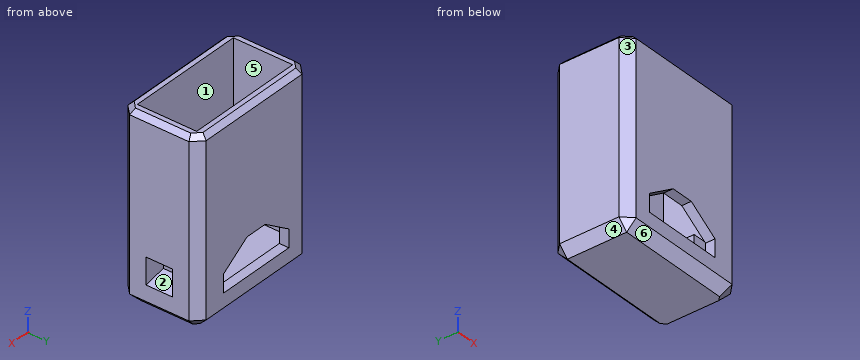
from build123d import *

# Parameters (mm, degrees)
F0_W      = 29
F0_H      = 16.5
F1_DEPTH  = 38.5
F2_T      = -2
F3_DEPTH  = 2.25
F4_SIZE   = 2
F5_SIZE   = 2
F6_SIZE   = 1
F8_DEPTH  = 16.501
F9_W      = 7.54
F9_H      = 7.25
F9_R      = 1.1
F10_DEPTH = 6.35
F11_W     = 5.538
F11_H     = 5.533
F13_W     = 5.538
F13_H     = 4.583


with BuildPart() as f1:
    # F0 (on Top) → F1 (new body)
    with BuildSketch(Plane.XY):
        with Locations((14.5, 8.25)):
            Rectangle(F0_W, F0_H)
    extrude(amount=F1_DEPTH)

    # F2
    f2_openings = [f1.faces().sort_by_distance(p)[0] for p in [
        (14.5, 8.25, 38.5),
    ]]
    offset(amount=F2_T, openings=f2_openings)

    # F3 (add): a face of the model
    f3_faces = [f1.faces().sort_by_distance(p)[0] for p in [
        (14.5, 8.25, 2),
    ]]
    extrude(f3_faces, amount=F3_DEPTH)

    # F4
    f4_edges = [f1.edges().sort_by_distance(p)[0] for p in [
        (29, 0, 19.25),
        (29, 16.5, 19.25),
    ]]
    chamfer(f4_edges, length=F4_SIZE)

    # F5
    f5_edges = [f1.edges().sort_by_distance(p)[0] for p in [
        (0, 16.5, 19.25),
        (0, 0, 19.25),
        (13.5, 16.5, 0),
        (13.5, 0, 0),
        (28, 1, 0),
        (0, 8.25, 0),
        (29, 8.25, 0),
        (28, 15.5, 0),
    ]]
    chamfer(f5_edges, length=F5_SIZE)

    # F6
    f6_edges = [f1.edges().sort_by_distance(p)[0] for p in [
        (0, 8.25, 38.5),
        (1, 1, 38.5),
        (14.5, 0, 38.5),
        (1, 15.5, 38.5),
        (14.5, 16.5, 38.5),
        (28, 15.5, 38.5),
        (29, 8.25, 38.5),
        (28, 1, 38.5),
    ]]
    chamfer(f6_edges, length=F6_SIZE)

    # F7 (on face) → F8 (cut, through all)
    with BuildSketch(Plane(origin=(0, 16.5, 0), x_dir=(-1, 0, 0), z_dir=(0, 1, 0))):
        Polygon((-22.536, 8.664), (-22.536, 4.94), (-5.464, 4.94), (-5.464, 8.664), (-11.635, 12.834), (-16.365, 12.834), align=None)
    extrude(amount=-F8_DEPTH, mode=Mode.SUBTRACT)

    # F9 (on face) → F10 (join)
    with BuildSketch(Plane.YZ.offset(29)):
        with Locations((8.25, 7.875)):
            Rectangle(F9_W, F9_H)
        with Locations((8.25, 9)):
            Circle(F9_R, mode=Mode.SUBTRACT)
    extrude(amount=-F10_DEPTH)

    # F11 (on face) → F14 section 0
    with BuildSketch(Plane.YZ.offset(29)):
        with Locations((8.25, 8.0385)):
            Rectangle(F11_W, F11_H)
    # F13 (on offset) → F14 section 1
    with BuildSketch(Plane.YZ.offset(24.55)):
        with Locations((8.25, 8.5135)):
            Rectangle(F13_W, F13_H)
    loft(mode=Mode.SUBTRACT)


solid = f1.part
Can you work these out from the model? Positions are in its coordinate system, mm. Face numbers are marked on the shaded views. A direction names the side the tool comes from. Coordinates: 2 decimals unless noted, no trailing zeros. Order: outer loops, then holes, each group sorted by start corner. A loop starts at its lowest first (then second) coordinate and runs counter-clockwise, first axis right, second up. Notation, with made-up numbers: (16, 12) -> (25, 12) arc R32 cw to (25, 49) -> close; hole circle Ø7 at (21.25, 21). An arc over 180 degrees is marked (long way). Use one line per item in the form item = value.
Q1. Imagine slicing it at A-A, the plane x = 14.25. List the corners of the cut face in (y, z) for me, then the cut area to 3 significant figures.
From the geometry:
outline = (0, 2) -> (2, 0) -> (14.5, 0) -> (16.5, 2) -> (16.5, 4.94) -> (14.5, 4.94) -> (14.5, 4.25) -> (2, 4.25) -> (2, 4.94) -> (0, 4.94) -> close; (0, 12.83) -> (2, 12.83) -> (2, 38.5) -> (1, 38.5) -> (0, 37.5) -> close; (14.5, 12.83) -> (16.5, 12.83) -> (16.5, 37.5) -> (15.5, 38.5) -> (14.5, 38.5) -> close
area = 171 mm²
Q2. I need wall thicknesses on L1, parallel to Y at x = 17, z = 4.5; L2, parallel to X at y = 11.25, z = 18.5; L3, parallel to Z at x = 23.2, y = 8.25. Which ranges of each line are inside material? Lowest first, please.
From the geometry:
L1 = 0 to 2, 14.5 to 16.5
L2 = 0 to 2, 27 to 29
L3 = 0 to 7.9, 10.1 to 11.5
Q3. Imagine slicing it at B-B, the plane y = 8.25. List the corners of the cut face in (x, z) for me (3 decimals).
From the geometry:
outline = (0, 2) -> (2, 0) -> (27, 0) -> (29, 2) -> (29, 5.272) -> (24.55, 6.222) -> (24.55, 7.9) -> (22.65, 7.9) -> (22.65, 4.25) -> (2, 4.25) -> (2, 38.5) -> (1, 38.5) -> (0, 37.5) -> close; (22.65, 10.1) -> (24.55, 10.1) -> (24.55, 10.805) -> (29, 10.805) -> (29, 37.5) -> (28, 38.5) -> (27, 38.5) -> (27, 11.5) -> (22.65, 11.5) -> close
Q4. Imagine slicing it at C-C, the plane z = 26. List the corners of the cut face in (x, y) for me.
From the geometry:
outline = (0, 2) -> (2, 0) -> (27, 0) -> (29, 2) -> (29, 14.5) -> (27, 16.5) -> (2, 16.5) -> (0, 14.5) -> close; hole (2, 2) -> (27, 2) -> (27, 14.5) -> (2, 14.5) -> close
Q5. Which directions (+Z, -Z, +X, -X, +Y, -Y) give clear straight access to the entire face, cutting with the end or side of a thin tool? Please do the marked faces 1, 2 and 3.
From the geometry:
face_1 = +Z
face_2 = +X
face_3 = +Z, -Z, -X, -Y
Q6. Imagine slicing it at D-D, the plane y = 3.75. List the corners of the cut face in (x, z) for me, then the cut area to 3 significant figures.
From the geometry:
outline = (0, 2) -> (2, 0) -> (27, 0) -> (29, 2) -> (29, 37.5) -> (28, 38.5) -> (27, 38.5) -> (27, 4.25) -> (2, 4.25) -> (2, 38.5) -> (1, 38.5) -> (0, 37.5) -> close
area = 255 mm²
Q7. We'd pull the mould along X, two halves only. Please class the marked faces 4, 5 and 6: released by +X, released by -X, zero draft, split by the parting line, or undercut.
From the geometry:
face_4 = released by -X
face_5 = undercut
face_6 = zero draft
Q8. Will these pins go through, and if not, where does the flat tip stop? P1, Ø1.3, axis at x = 25.5, y = 7.5, coming from the +Z side; P2, Ø1.3, axis at x = 27.5, y = 8.5, coming from the -Z side; P3, Ø2.5, axis at y = 8.25, z = 9, coming from the +X side; P4, Ø2, axis at y = 16, z = 7, coming from the -X side.
From the geometry:
P1 = 11.5
P2 = 0
P3 = 24.55
P4 = 0.5
